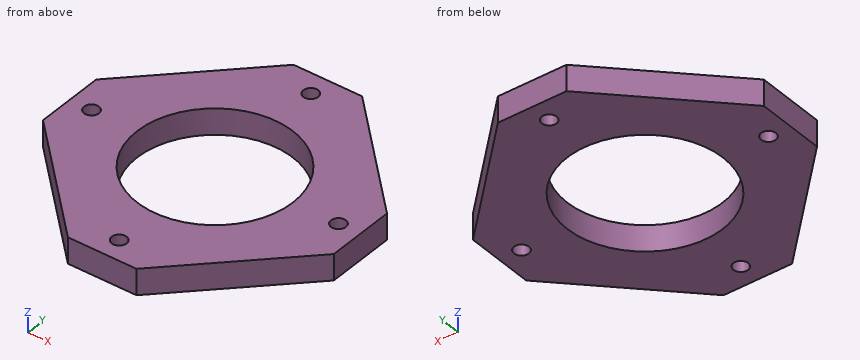
```python
from build123d import *

# Parameters (mm, degrees)
SKETCH1_W           = 78.5
SKETCH1_H           = 78.5
BOSS_EXTRUDE1_DEPTH = 3.5
SKETCH3_R           = 21
CUT_EXTRUDE2_DEPTH  = 56.947520052
SKETCH4_R           = 2
CUT_EXTRUDE3_DEPTH  = 56.947520052
CHAMFER1_SIZE       = 30


with BuildPart() as part:
    # Sketch1 → Boss-Extrude1 (new, symmetric)
    with BuildSketch(Plane.XY):
        Rectangle(SKETCH1_W, SKETCH1_H)
    extrude(amount=BOSS_EXTRUDE1_DEPTH, both=True)

    # Sketch3 → Cut-Extrude2 (cut, through all)
    with BuildSketch(Plane.XY.offset(3.5)):
        Circle(SKETCH3_R)
    extrude(amount=-CUT_EXTRUDE2_DEPTH, mode=Mode.SUBTRACT)

    # Sketch4 → Cut-Extrude3 (cut, through all)
    with BuildSketch(Plane.XY.offset(3.5)):
        with Locations((0, 33.333013665)):
            Circle(SKETCH4_R)
        with Locations((-33.333013665, 0)):
            Circle(SKETCH4_R)
        with Locations((0, -33.333013665)):
            Circle(SKETCH4_R)
        with Locations((33.333013665, 0)):
            Circle(SKETCH4_R)
    extrude(amount=-CUT_EXTRUDE3_DEPTH, mode=Mode.SUBTRACT)

    # Chamfer1
    chamfer1_edges = [part.edges().sort_by_distance(p)[0] for p in [
        (39.25, -39.25, 0),
        (-39.25, -39.25, 0),
        (-39.25, 39.25, 0),
        (39.25, 39.25, 0),
    ]]
    chamfer(chamfer1_edges, length=CHAMFER1_SIZE)


solid = part.part
```
Verification items for the finished model (mm, model axes). Round coordinates to 2 decimals unless told otherwise and drop trailing zeros. Order: outer loops, then holes, each group sorted by start corner. A loop starts at its lowest first (then second) coordinate and runs counter-clockwise, first axis right, second up. Notation, with made-up numbers: (-28, 50) -> (19, 50) arc R28 ccw to (19, 68) -> close; hole circle Ø9 at (28.25, -36.5). An arc over 180 degrees is marked (long way). Put each result on its own line as item: value. Start each with the question number.
(1) Material ranges on line 1 along Y through (x, z) = (0, 1); line 2 along Y through (x, z) = (-0.5, -2); line 3 along X through (y, z) = (1.5, 1), recorded low to high.
(2) Depth check by flat-ended pin: pin 1 Ø2 at (x, z) = (23, 0.5) entering from +Y. Enter the tip coordinate at first touch or a pass-through.
(3) Section check A-A (x = 0). Enter the section's corners in (y, z), then the cut area to 4 significant figures.
(4) Section check D-D (z = 0.5). Enter the section's corners in (x, y), then the cut area to 3 significant figures.
(5) Section check C-C (y = -17.5). Enter the section's corners in (x, z), then the cut area to 3 significant figures.
Completed:
1. line 1: y = -39.25 to -35.33, -31.33 to -21, 21 to 31.33, 35.33 to 39.25
1. line 2: y = -39.25 to -35.27, -31.4 to -20.99, 20.99 to 31.4, 35.27 to 39.25
1. line 3: x = -39.25 to -34.66, -32.01 to -20.95, 20.95 to 32.01, 34.66 to 39.25
2. pin 1: stops at y = 26.5
3. outline: (-39.25, -3.5) -> (-35.33, -3.5) -> (-35.33, 3.5) -> (-39.25, 3.5) -> close; (-31.33, -3.5) -> (-21, -3.5) -> (-21, 3.5) -> (-31.33, 3.5) -> close; (21, -3.5) -> (31.33, -3.5) -> (31.33, 3.5) -> (21, 3.5) -> close; (35.33, -3.5) -> (39.25, -3.5) -> (39.25, 3.5) -> (35.33, 3.5) -> close
3. area: 199.5 mm2
4. outline: (-39.25, -9.25) -> (-9.25, -39.25) -> (9.25, -39.25) -> (39.25, -9.25) -> (39.25, 9.25) -> (9.25, 39.25) -> (-9.25, 39.25) -> (-39.25, 9.25) -> close; hole circle Ø4 at (-33.33, 0); hole circle Ø42 at (0, 0); hole circle Ø4 at (0, -33.33); hole circle Ø4 at (0, 33.33); hole circle Ø4 at (33.33, 0)
4. area: 2,930 mm2
5. outline: (-31, -3.5) -> (-11.61, -3.5) -> (-11.61, 3.5) -> (-31, 3.5) -> close; (11.61, -3.5) -> (31, -3.5) -> (31, 3.5) -> (11.61, 3.5) -> close
5. area: 271 mm2
